Can you work these out from the model? Positions are in its coordinate system, mm. A direction names the side the tool comes from. Coordinates: 2 decimals unless noted, no trailing zeros. Order: outer loops, then holes, each group sorted by start corner. A loop starts at its lowest first (then second) coordinate and runs counter-clockwise, first axis right, second up. Notation, with made-up numbers: (20.5, 81.25) -> (55.5, 81.25) arc R13 cw to (55.5, 92.25) -> close; hole circle Ø1 at (-5, 44.5). An arc over 180 degrees is marked (long way). Answer as CSV lines item,"result".
Autodesk Inventor part; units mm, degrees
ref_plane "YZ Plane" through (0, 0, 0) normal (1, 0, 0) x (0, 1, 0)
ref_plane "XZ Plane" through (0, 0, 0) normal (0, 1, 0) x (-1, 0, 0)
ref_plane "XY Plane" through (0, 0, 0) normal (0, 0, 1) x (1, 0, 0)
sketch "Sketch1" plane through (0, 0, 0) normal (1, 0, 0) x (0, 1, 0)
  line L0 (0, 0) -> (-25.4, 0)
  line L1 (-25.4, 0) -> (-25.4, 25.4)
  line L2 (-25.4, 25.4) -> (0, 25.4)
  line L3 (0, 25.4) -> (0, 0)
  line L4 (-3.175, 3.175) -> (-22.225, 3.175)
  line L5 (-22.225, 3.175) -> (-22.225, 22.225)
  line L6 (-22.225, 22.225) -> (-3.175, 22.225)
  line L7 (-3.175, 22.225) -> (-3.175, 3.175)
  dimension "d0" = 25.4
  dimension "d1" = 25.4
  dimension "d2" = 19.05
  dimension "d3" = 19.05
  dimension "d4" = 3.175
  dimension "d5" = 3.175
extrude "Extrusion1" add sketch "Sketch1" along normal blind 546.1
sketch "Sketch2" plane through (0, -25.4, 25.4) normal (0, 0, 1) x (1, 0, 0)
  line L0 (0, 0) -> (0, 25.4)
  line L1 (0, 0) -> (546.1, 0)
  line L2 (546.1, 25.4) -> (546.1, 0)
  line L3 (0, 25.4) -> (546.1, 25.4)
  point P0 (12.7, 12.7)
  point P1 (533.4, 12.7)
  dimension "d8" = 12.7
  dimension "d9" = 12.7
  dimension "d10" = 12.7
  dimension "d11" = 12.7
hole "Hole1" at (12.7, -12.7, 25.4) at (533.4, -12.7, 25.4) direction (0, 0, -1) diameter 6.35 end through all
sketch "Sketch3" plane through (0, -25.4, 25.4) normal (0, 0, 1) x (1, 0, 0)
  circle A0 centre (12.7, 12.7) radius 3.175
  circle A1 centre (533.4, 12.7) radius 3.175
  line L0 (0, 0) -> (0, 25.4)
  line L1 (0, 0) -> (546.1, 0)
  line L2 (546.1, 25.4) -> (546.1, 0)
  line L3 (0, 25.4) -> (546.1, 25.4)
  point P0 (247.65, 12.7)
  point P1 (298.45, 12.7)
  dimension "d19" = 247.65
  dimension "d20" = 247.65
  dimension "d21" = 12.7
  dimension "d22" = 12.7
hole "Hole2" at (247.65, -12.7, 25.4) at (298.45, -12.7, 25.4) direction (0, 0, -1) diameter 6.35 end through all
sketch "Sketch4" plane through (0, -25.4, 25.4) normal (0, 0, 1) x (1, 0, 0)
  circle A0 centre (247.65, 12.7) radius 3.175
  circle A1 centre (298.45, 12.7) radius 3.175
  circle A2 centre (12.7, 12.7) radius 3.175
  circle A3 centre (533.4, 12.7) radius 3.175
  line L0 (0, 0) -> (0, 25.4)
  line L1 (0, 0) -> (546.1, 0)
  line L2 (546.1, 25.4) -> (546.1, 0)
  line L3 (0, 25.4) -> (546.1, 25.4)
  point P0 (38.1, 12.7)
  point P1 (508, 12.7)
  dimension "d30" = 38.1
  dimension "d31" = 12.7
  dimension "d32" = 12.7
  dimension "d33" = 38.1
hole "Hole3" at (38.1, -12.7, 25.4) at (508, -12.7, 25.4) direction (0, 0, -1) diameter 4.7625 end through all
sketch "Sketch7" plane through (0, -25.4, 25.4) normal (0, 0, 1) x (1, 0, 0)
  circle A0 centre (38.1, 12.7) radius 2.3813
  circle A1 centre (508, 12.7) radius 2.3813
  line L0 (0, 0) -> (546.1, 0)
  circle A2 centre (38.1, 12.7) radius 3.175
  circle A3 centre (95.25, 12.7) radius 3.175
  circle A4 centre (508, 12.7) radius 2.3813
  circle A5 centre (508, 12.7) radius 3.175
  circle A6 centre (450.85, 12.7) radius 3.175
  dimension "d65" = 6.35
  dimension "d66" = 6.35
  dimension "d67" = 12.7
  dimension "d68" = 57.15
  dimension "d69" = 6.35
  dimension "d70" = 6.35
  dimension "d71" = 12.7
  dimension "d72" = 57.15
extrude "Extrusion2" cut sketch "Sketch7" against normal blind 25.4
sketch "Sketch8" plane through (0, 0, 0) normal (-1, 0, 0) x (0, 0, 1)
  line L0 (22.225, -22.225) -> (3.175, -22.225)
  line L1 (3.175, -22.225) -> (3.175, -3.175)
  line L2 (3.175, -3.175) -> (22.225, -3.175)
  line L3 (22.225, -3.175) -> (22.225, -22.225)
  line L4 (0, 0) -> (0, -25.4)
  line L5 (0, -25.4) -> (25.4, -25.4)
  line L6 (25.4, -25.4) -> (25.4, 0)
  line L7 (25.4, 0) -> (0, 0)
extrude "Extrusion3" cut sketch "Sketch8" against normal blind 25.4
sketch "Sketch9" plane through (546.1, 0, 0) normal (1, 0, 0) x (0, 0, -1)
  line L0 (-3.175, -22.225) -> (-22.225, -22.225)
  line L1 (-22.225, -22.225) -> (-22.225, -3.175)
  line L2 (-22.225, -3.175) -> (-3.175, -3.175)
  line L3 (-3.175, -3.175) -> (-3.175, -22.225)
  line L4 (0, -25.4) -> (0, 0)
  line L5 (0, 0) -> (-25.4, 0)
  line L6 (-25.4, 0) -> (-25.4, -25.4)
  line L7 (-25.4, -25.4) -> (0, -25.4)
extrude "Extrusion4" cut sketch "Sketch9" against normal blind 25.4
properties part number "1x1 horizontal support" material "Aluminum 6061"
Q1. We'd pull the mould along Y, two halves only. Please class faces 1 (the flat face through (25.4, -13, 24)), 2 (the flat face through (270, -25.4, 13)), 3 (the flat face through (270, -22.225, 13)): pulls with the +Y half, pulls with the -Y half, needs draft (parallel to the pull), parting line crosses it, or undercut.
Solution:
face 1,"needs draft"
face 2,"pulls with the -Y half"
face 3,"undercut"
Q2. Imagine slicing it at A-A (x = 233). List the corners of the cut face in (y, z) for me (3 decimals).
Solution:
outline,"(-25.4, 0) -> (0, 0) -> (0, 25.4) -> (-25.4, 25.4) -> close; hole (-22.225, 3.175) -> (-3.175, 3.175) -> (-3.175, 22.225) -> (-22.225, 22.225) -> close"
Q3. Which directions (+Z, -Z, +X, -X, +Y, -Y) give clear straight access to the entire face, cutting with the end or side of a thin tool? Please do faces 4 (the flat face through (270, -13, 0)), 5 (the flat face through (270, -13, 22.225)).
Solution:
face 4,"-Z, +X, -X, +Y, -Y"
face 5,"+X, -X"
Q4. If I drill on line 1 (Z direction, x = 217, y = -5.25) (3 decimals); line 2 (Y direction, x = 247.65, z = 1.5) (3 decimals); line 3 (Y direction, x = 140.5, z = 7.25) (3 decimals), over which ranges is the centre line in solid material (lowest first)?
Solution:
line 1,"0 to 3.175, 22.225 to 25.4"
line 2,"-25.4 to -15.875, -9.525 to 0"
line 3,"-25.4 to -22.225, -3.175 to 0"
Q5. Imagine slicing it at B-B (z = 18). List the corners of the cut face in (x, y) for me (3 decimals).
Solution:
outline,"(25.4, -25.4) -> (520.7, -25.4) -> (520.7, -22.225) -> (25.4, -22.225) -> close; (25.4, -3.175) -> (520.7, -3.175) -> (520.7, 0) -> (25.4, 0) -> close"
Q6. For P1, Ø10, axis at x = 101.5, z = 21, coming from the +Y side, with a flat end and sliding along its axis, tell me the tip position at first contact or that it passes through.
Solution:
P1,"y = 0"
